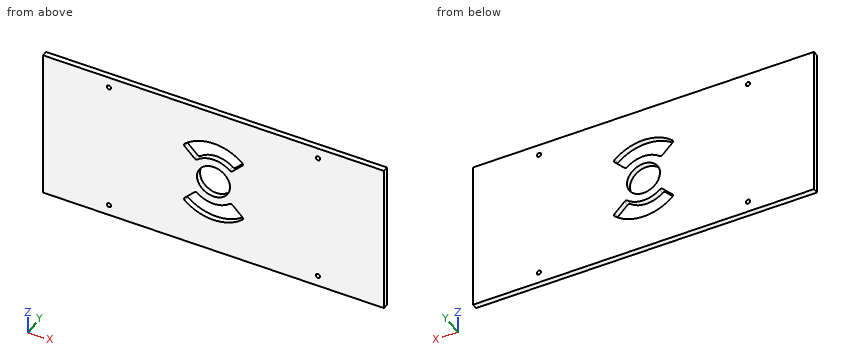
from build123d import *

# Parameters (mm, degrees)
SKETCH2_W           = 310
SKETCH2_H           = 140
BOSS_EXTRUDE1_DEPTH = 5
SKETCH3_R           = 15
CUT_EXTRUDE1_DEPTH  = 171.146995272
SKETCH5_R           = 2
CUT_EXTRUDE2_DEPTH  = 171.146995272
CUT_EXTRUDE3_DEPTH  = 10
FILLET1_R           = 2


with BuildPart() as part:
    # Sketch2 → Boss-Extrude1 (new body)
    with BuildSketch(Plane(origin=(0, 0, 0), x_dir=(1, 0, 0), z_dir=(0, 1, 0))):
        Rectangle(SKETCH2_W, SKETCH2_H)
    extrude(amount=BOSS_EXTRUDE1_DEPTH)

    # Sketch3 → Cut-Extrude1 (cut, through all)
    with BuildSketch(Plane(origin=(0, 5, 0), x_dir=(1, 0, 0), z_dir=(0, 1, 0))):
        with Locations(Location((0, 0, 0), (0, 0, 270))):
            Circle(SKETCH3_R)
    extrude(amount=-CUT_EXTRUDE1_DEPTH, mode=Mode.SUBTRACT)

    # Sketch5 → Cut-Extrude2 (cut, through all)
    with BuildSketch(Plane(origin=(0, 5, 0), x_dir=(1, 0, 0), z_dir=(0, 1, 0))):
        with Locations(Location((-95, 60, 0), (0, 0, 270))):
            Circle(SKETCH5_R)
        with Locations(Location((95, 60, 0), (0, 0, 90))):
            Circle(SKETCH5_R)
        with Locations(Location((95, -60, 0), (0, 0, 270))):
            Circle(SKETCH5_R)
        with Locations(Location((-95, -60, 0), (0, 0, 90))):
            Circle(SKETCH5_R)
    extrude(amount=-CUT_EXTRUDE2_DEPTH, mode=Mode.SUBTRACT)

    # Sketch6 → Cut-Extrude3 (cut)
    with BuildSketch(Plane(origin=(0, 5, 0), x_dir=(1, 0, 0), z_dir=(0, 1, 0))):
        with BuildLine():
            Line((27.577164466, -27.577164466), (15.909902577, -15.909902577))
            ThreePointArc((15.909902577, -15.909902577), (0, -22.5), (-15.909902577, -15.909902577))
            Line((-15.909902577, -15.909902577), (-27.577164466, -27.577164466))
            ThreePointArc((-27.577164466, -27.577164466), (0, -39), (27.577164466, -27.577164466))
        make_face()
        with BuildLine():
            ThreePointArc((-15.909902577, 15.909902577), (0, 22.5), (15.909902577, 15.909902577))
            Line((15.909902577, 15.909902577), (27.577164466, 27.577164466))
            ThreePointArc((27.577164466, 27.577164466), (0, 39), (-27.577164466, 27.577164466))
            Line((-27.577164466, 27.577164466), (-15.909902577, 15.909902577))
        make_face()
    extrude(amount=-CUT_EXTRUDE3_DEPTH, mode=Mode.SUBTRACT)

    # Fillet1
    fillet1_edges = [part.edges().sort_by_distance(p)[0] for p in [
        (-15.909902577, 2.5, 15.909902577),
        (15.909902577, 2.5, 15.909902577),
        (27.577164466, 2.5, 27.577164466),
        (-27.577164466, 2.5, 27.577164466),
        (15.909902577, 2.5, -15.909902577),
        (-15.909902577, 2.5, -15.909902577),
        (-27.577164466, 2.5, -27.577164466),
        (27.577164466, 2.5, -27.577164466),
    ]]
    fillet(fillet1_edges, radius=FILLET1_R)


solid = part.part
Could you check a few things on this model? Use its own coordinates, in mm. Give positions to 0.01 mm unless a question says otherwise; leave off trailing zeros. Order: outer loops, then holes, each group sorted by start corner. A loop starts at its lowest first (then second) coordinate and runs counter-clockwise, first axis right, second up.
1. Suppose I cut it at B-B (y = 1.85). Write out the boundary of the cut face in (x, z), plus the area to 3 significant figures.
Answers below:
outline: (-155, -70) - (155, -70) - (155, 70) - (-155, 70) - close; hole circle Ø4 at (-95, -60); hole circle Ø4 at (-95, 60); hole (-26.12, -26.12) arc R2 ccw to (-26.05, -29.03) arc R39 ccw to (26.05, -29.03) arc R2 ccw to (26.12, -26.12) - (17.27, -17.27) arc R2 ccw to (14.56, -17.16) arc R22.5 cw to (-14.56, -17.16) arc R2 ccw to (-17.27, -17.27) - close; hole (-26.12, 26.12) - (-17.27, 17.27) arc R2 ccw to (-14.56, 17.16) arc R22.5 cw to (14.56, 17.16) arc R2 ccw to (17.27, 17.27) - (26.12, 26.12) arc R2 ccw to (26.05, 29.03) arc R39 ccw to (-26.05, 29.03) arc R2 ccw to start; hole circle Ø30 at (0, 0); hole circle Ø4 at (95, -60); hole circle Ø4 at (95, 60)
area: 41,100 mm2
2. I need wall thicknesses on L1, parallel to X at y = 2.15, z = 60; L2, parallel to X at y = 1.8, z = 19.5; L3, parallel to X at y = 1.8, z = 3. Which ranges of each line are inside material? Lowest first, please.
Answers below:
L1: x = -155 to -97, -93 to 93, 97 to 155
L2: x = -155 to -19.5, -11.22 to 11.22, 19.5 to 155
L3: x = -155 to -14.7, 14.7 to 155
3. Suppose I cut it at C-C (x = 0). Write out the boundary of the cut face in (y, z).
Answers below:
outline: (0, -70) - (5, -70) - (5, -39) - (0, -39) - close; (0, -22.5) - (5, -22.5) - (5, -15) - (0, -15) - close; (0, 15) - (5, 15) - (5, 22.5) - (0, 22.5) - close; (0, 39) - (5, 39) - (5, 70) - (0, 70) - close
4. Suppose I cut it at A-A (z = 0). Write out the boundary of the cut face in (x, y), plus the area to 3 significant figures.
Answers below:
outline: (-155, 0) - (-15, 0) - (-15, 5) - (-155, 5) - close; (15, 0) - (155, 0) - (155, 5) - (15, 5) - close
area: 1,400 mm2
